from build123d import *

# Parameters (mm, degrees)
F1_DEPTH = 16
F2_R     = 6.5
F3_DEPTH = 36.5
F4_R     = 5.5
F5_DEPTH = 13
F6_SIZE  = 10


with BuildPart() as f1:
    # F0 (on Front) → F1 (new body, symmetric)
    with BuildSketch(Plane.XZ):
        Polygon((-56.5, 13), (-56.5, 0), (-17.5, 0), (-17.5, 17), (17.5, 17), (17.5, 0), (56.5, 0), (56.5, 13), (31.5, 13), (31.5, 64), (12.5, 64), (12.5, 30), (-12.5, 30), (-12.5, 64), (-31.5, 64), (-31.5, 13), align=None)
    extrude(amount=F1_DEPTH, both=True)

    # F2 (on Right) → F3 (cut, symmetric)
    with BuildSketch(Plane.YZ):
        with Locations((0, 46)):
            Circle(F2_R)
    extrude(amount=F3_DEPTH, both=True, mode=Mode.SUBTRACT)

    # F4 (on Top) → F5 (cut)
    with BuildSketch(Plane.XY):
        with Locations((-43.5, 3)):
            Circle(F4_R)
        with Locations((43.5, 3)):
            Circle(F4_R)
    extrude(amount=F5_DEPTH, mode=Mode.SUBTRACT)

    # F6
    f6_edges = [f1.edges().sort_by_distance(p)[0] for p in [
        (56.5, -16, 6.5),
        (-56.5, -16, 6.5),
    ]]
    chamfer(f6_edges, length=F6_SIZE)


solid = f1.part
Source: CAD feature listing. Evaluate the final solid. Frame: model axes, mm. A direction names the side the tool comes from. Coordinates: 2 decimals unless noted, no trailing zeros. Order: outer loops, then holes, each group sorted by start corner. A loop starts at its lowest first (then second) coordinate and runs counter-clockwise, first axis right, second up. Notation, with made-up numbers: M -5.5,-25.5 L 33.5,-25.5 A36 ccw 33.5,10.5 Z; hole C 75.5,47 d8. An arc over 180 degrees is marked long. Write each question's results on one line, items separated by ' | '. Start each with the question number.
1. Section D-D, the plane z = 46. Return the cut outline in (x, y), then the cut area to 3 significant figures.
2. Section A-A, the plane z = 54. Return the cut outline in (x, y).
3. Reachability of faces 1 (the face through (0, 0, 30)), 2 (the face through (-17.5, 0, 8)), 3 (the face through (44, -4, 13)) from +Z, -Z, +X, -X, +Y, -Y: full face, straight path, thin tool, end or side. Return the list, or none.
4. Pin query (flat end, axial travel): pin 1 (12.5 mm diameter, centred on x = 40.5, y = -2.5, fed in from +Z); pin 2 (16 mm diameter, centred on y = 3, z = 36.5, fed in from -X); pin 3 (1 mm diameter, centred on y = 5, z = 34.5, fed in from +X). Return the tip coordinate at first contact, or that it passes through.
5. Material intervals for L1, parallel to Y at x = 43.5, z = 10.25; L2, parallel to Z at x = -23.5, y = 0; L3, parallel to X at y = -9, z = 38.5, sorted ascending.
6. Section C-C, the plane y = 0. State how many separate pieces and enclosed holes the cut face has, then the cut area to 3 significant figures.
7. Section B-B, the plane x = -43.5. Return the cut outline in (y, z).
8. Draft query along Y for faces 4 (the face through (-21.867, -1.409, 39.655)), 5 (the face through (-31.5, 0, 39)), 6 (the face through (10, -16, 25)). Return one class per face: +Y half, -Y half, draft (parallel to the pull), parting line (faces both ways), or undercut.
Solution:
1) outline: M -31.5,-16 L -12.5,-16 L -12.5,-6.5 L -31.5,-6.5 Z; M -31.5,6.5 L -12.5,6.5 L -12.5,16 L -31.5,16 Z; M 12.5,-16 L 31.5,-16 L 31.5,-6.5 L 12.5,-6.5 Z; M 12.5,6.5 L 31.5,6.5 L 31.5,16 L 12.5,16 Z | area: 722 mm²
2) outline: M -31.5,-16 L -12.5,-16 L -12.5,16 L -31.5,16 Z; M 12.5,-16 L 31.5,-16 L 31.5,16 L 12.5,16 Z
3) face 1: +Z, +Y, -Y | face 2: -Z, +Y, -Y | face 3: +Z, +X, +Y, -Y
4) pin 1: z = 13 | pin 2: x = -31.5 | pin 3: x = 31.5
5) L1: -16 to -2.5, 8.5 to 16 | L2: 0 to 39.5, 52.5 to 64 | L3: -31.5 to -12.5, 12.5 to 31.5
6) separate pieces: 5 | enclosed holes: 0 | area: 2,500 mm²
7) outline: M -16,0 L -2.5,0 L -2.5,13 L -16,13 Z; M 8.5,0 L 16,0 L 16,13 L 8.5,13 Z
8) face 4: undercut | face 5: draft | face 6: -Y half
